Geometry check sheet. Reference: the model listing, model coordinates, mm. A direction names the side the tool comes from. Give positions to 0.01 mm unless a question says otherwise; leave off trailing zeros. Loops run counter-clockwise (first coordinate to the right, second up) from the corner with the lowest first, then second, coordinate; pieces in that order, holes last. Notation, with made-up numbers: (18.25, 72.5) -> (26.25, 72.5) arc R24 ccw to (26.25, 106.5) -> close; hole circle Ø10 at (65, 56). An arc over 180 degrees is marked (long way). One line per question, with ' | ' between items.
from build123d import *

# Parameters (mm, degrees)
SKETCH1_W           = 47
SKETCH1_H           = 62
SKETCH1_R           = 1.75
BOSS_EXTRUDE1_DEPTH = 1.6
BOSS_EXTRUDE2_DEPTH = 12


with BuildPart() as part:
    # Sketch1 → Boss-Extrude1 (new body)
    with BuildSketch(Plane(origin=(0, 0, 0), x_dir=(1, 0, 0), z_dir=(0, 1, 0))):
        Rectangle(SKETCH1_W, SKETCH1_H)
        with Locations(Location((-20.5, -28, 0), (0, 0, 270))):
            Circle(SKETCH1_R, mode=Mode.SUBTRACT)
        with Locations(Location((20.5, -28, 0), (0, 0, 270))):
            Circle(SKETCH1_R, mode=Mode.SUBTRACT)
        with Locations(Location((20.5, 28, 0), (0, 0, 270))):
            Circle(SKETCH1_R, mode=Mode.SUBTRACT)
        with Locations(Location((-20.5, 28, 0), (0, 0, 270))):
            Circle(SKETCH1_R, mode=Mode.SUBTRACT)
    extrude(amount=-BOSS_EXTRUDE1_DEPTH)

    # Sketch3 → Boss-Extrude2 (add)
    with BuildSketch(Plane(origin=(0, 0, 0), x_dir=(1, 0, 0), z_dir=(0, 1, 0))):
        Polygon((-22.5, 22), (-17.9, 22), (-17.9, 29.7), (17.5, 29.7), (17.5, 22), (20.5, 22), (20.5, -24), (-22.5, -24), align=None)
    extrude(amount=BOSS_EXTRUDE2_DEPTH)


solid = part.part
Item 1: Release check for a two-part mould opening along X. For faces 4 (the face through (-17.9, 6, -26)), 5 (the face through (-19.32, -0.79, -29.29)), 6 (the face through (0, -1, 31)) record: pulls with the +X half, pulls with the -X half, needs draft (parallel to the pull), parting line crosses it, or undercut.
Result:
face 4: pulls with the -X half | face 5: undercut | face 6: needs draft
Item 2: Set-up check for faces 1 (the face through (17.5, 6, -26)), 2 (the face through (-22.5, 6, 1)), 3 (the face through (20.5, 6, 1)): record each of +Z, -Z, +X, -X, +Y, -Y from which the full face is reachable in a straight line by a thin tool's end or side.
Result:
face 1: -Z, +X, +Y | face 2: +Z, -Z, -X, +Y | face 3: +Z, -Z, +X, +Y
Item 3: Depth check by flat-ended pin: pin 1 Ø0.9 at (x, y) = (19, 4.5) entering from -Z; pin 2 Ø1 at (x, y) = (-9.5, 2.5) entering from -Z; pin 3 Ø6 at (y, z) = (5, -26.5) entering from +X. Enter the tip coordinate at first touch or a pass-through.
Result:
pin 1: z = -22 | pin 2: z = -29.7 | pin 3: x = 17.5
Item 4: Sectioned sample at A-A (z = -28). Record the cut outline in (x, y), plus the area to 3 significant figures.
Result:
outline: (-23.5, -1.6) -> (-22.25, -1.6) -> (-22.25, 0) -> (-23.5, 0) -> close; (-18.75, -1.6) -> (18.75, -1.6) -> (18.75, 0) -> (17.5, 0) -> (17.5, 12) -> (-17.9, 12) -> (-17.9, 0) -> (-18.75, 0) -> close; (22.25, -1.6) -> (23.5, -1.6) -> (23.5, 0) -> (22.25, 0) -> close | area: 489 mm2
Item 5: Sectioned sample at B-B (x = -13). Record the cut outline in (y, z), plus the area to 3 significant figures.
Result:
outline: (-1.6, -31) -> (0, -31) -> (0, -29.7) -> (12, -29.7) -> (12, 24) -> (0, 24) -> (0, 31) -> (-1.6, 31) -> close | area: 744 mm2
Item 6: Sectioned sample at D-D (z = -19.5). Record the cut outline in (x, y).
Result:
outline: (-23.5, -1.6) -> (23.5, -1.6) -> (23.5, 0) -> (20.5, 0) -> (20.5, 12) -> (-22.5, 12) -> (-22.5, 0) -> (-23.5, 0) -> close
Item 7: Scan lines: probe 1 along X at (y, z) = (-0.5, -28); probe 2 along X at (y, z) = (4.5, 20); probe 3 along Z at (x, y) = (7, 11). Record each from-to range of solid material in increasing order.
Result:
probe 1: -23.5 to -22.25, -18.75 to 18.75, 22.25 to 23.5 | probe 2: -22.5 to 20.5 | probe 3: -29.7 to 24
Item 8: Sectioned sample at C-C (x = -20.5). Record the cut outline in (y, z), plus the area to 3 significant figures.
Result:
outline: (-1.6, -31) -> (0, -31) -> (0, -29.75) -> (-1.6, -29.75) -> close; (-1.6, -26.25) -> (0, -26.25) -> (0, -22) -> (12, -22) -> (12, 24) -> (0, 24) -> (0, 26.25) -> (-1.6, 26.25) -> close; (-1.6, 29.75) -> (0, 29.75) -> (0, 31) -> (-1.6, 31) -> close | area: 640 mm2
